Check sheet for the modelled part. Datum: model origin and axes. Units: mm. Face numbers are marked on the shaded views. A direction names the side the tool comes from. Round coordinates to 2 decimals unless told otherwise and drop trailing zeros. Order: outer loops, then holes, each group sorted by start corner. A loop starts at its lowest first (then second) coordinate and runs counter-clockwise, first axis right, second up. Notation, with made-up numbers: M 88,25.5 L 117,25.5 A19 ccw 117,47.5 Z; hole C 89,38 d10. An arc over 180 degrees is marked long. One line per item, written item: value. Start each with the question number.
(1) Cross-section at B-B, the plane y = 16. Enter the section's corners in (x, z).
(2) Release check for a two-part mould opening along Z. For the marked faces 1, 2, 3 and 4 record: released by +Z, released by -Z, zero draft, split by the parting line, or undercut.
(3) Access from +Z, -Z, +X, -X, +Y, -Y to the whole of each face (thin tool, end or side, straight path). Record for the marked faces 5, 6 and 7.
(4) Depth check by flat-ended pin: pin 1 Ø4 at (x, y) = (3, 14) entering from +Z; pin 2 Ø8 at (x, y) = (4.5, 14.5) entering from +Z. Enter the tip coordinate at first touch or a pass-through.
(5) Cross-section at A-A, the plane z = -41. Enter the section's corners in (x, y), and give its area (3 significant figures).
(6) Cross-section at C-C, the plane z = -18. Enter the section's corners in (x, y), and give its area (3 significant figures).
(7) Cross-section at D-D, the plane x = 3. Enter the section's corners in (y, z), and give its area (3 significant figures).
(8) Thickness scan on L1, parallel to X at y = 10, z = -40; L2, parallel to Y at x = -1.5, z = -62; L3, parallel to X at y = 13, z = -3. Record the ranges inside material, lowest first.
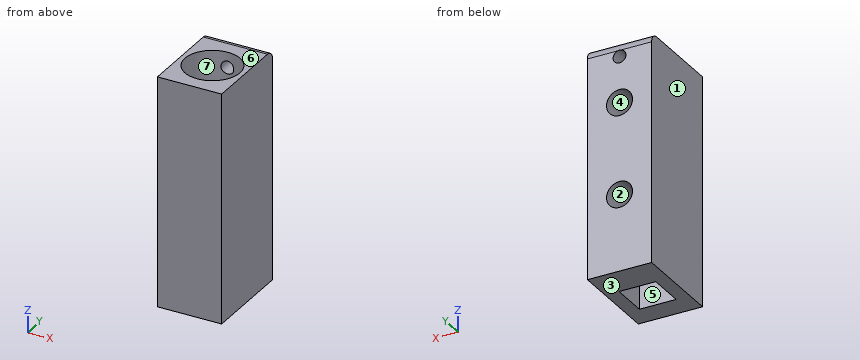
from build123d import *

# Parameters (mm, degrees)
SKETCH_1_W               = 21
SKETCH_1_H               = 30
EXTRUDE_1_DEPTH          = 75
CUT_EXTRUDE_1_DEPTH      = 82.457043894
CUT_EXTRUDE_1_DEPTH_BACK = 11
SKETCH_2_R               = 9
SKETCH_3_W               = 12
SKETCH_3_H               = 12
CUT_EXTRUDE_2_DEPTH      = 72.45802964
FILLET_1_R               = 3
HOLE_WIZARD_M5_1_REACH   = 83.457
HOLE_WIZARD_M5_1_BORE_R  = 2.1
HOLE_WIZARD_M10_1_D      = 8.5
HOLE_WIZARD_M10_1_DEPTH  = 10.5


with BuildPart() as part:
    # 草图1 → 凸台-拉伸1 (new body)
    with BuildSketch(Plane.XY):
        with Locations((0, 15)):
            Rectangle(SKETCH_1_W, SKETCH_1_H)
    extrude(amount=-EXTRUDE_1_DEPTH)

    # 草图2 → 切除-拉伸1 (cut, two sides: drawn at the far end of the back side and taken through both)
    with BuildSketch(Plane.XY.offset(-CUT_EXTRUDE_1_DEPTH_BACK)):
        with Locations(Location((0, 13.5, 0), (0, 0, 180))):
            Circle(SKETCH_2_R)
    extrude(amount=CUT_EXTRUDE_1_DEPTH + CUT_EXTRUDE_1_DEPTH_BACK, mode=Mode.SUBTRACT)

    # 草图3 → 切除-拉伸2 (cut, through all)
    with BuildSketch(Plane.XY.offset(-11)):
        with Locations((0, 13.5)):
            Rectangle(SKETCH_3_W, SKETCH_3_H)
    extrude(amount=-CUT_EXTRUDE_2_DEPTH, mode=Mode.SUBTRACT)

    # 圆角1
    fillet_1_edges = [part.edges().sort_by_distance(p)[0] for p in [
        (0, 30, 0),
    ]]
    fillet(fillet_1_edges, radius=FILLET_1_R)

    # M5 螺纹孔1 bore → M5 螺纹孔1 (cut, up to next)
    with BuildSketch(Plane(origin=(0, 30, 0), x_dir=(1, 0, 0), z_dir=(0, 1, 0)), mode=Mode.PRIVATE) as hole_wizard_m5_1_sk1:
        with Locations((0, 5)):
            Circle(HOLE_WIZARD_M5_1_BORE_R)
    hole_wizard_m5_1_tool1 = extrude(hole_wizard_m5_1_sk1.sketch, amount=-HOLE_WIZARD_M5_1_REACH, mode=Mode.PRIVATE) & part.part
    add(hole_wizard_m5_1_tool1.solids().sort_by_distance((0, 30, -5))[0], mode=Mode.SUBTRACT)

    # M10 螺纹孔1
    with Locations(Plane(origin=(0, 30, 0), x_dir=(1, 0, 0), z_dir=(0, 1, 0))):
        with Locations((0, 20), (0, 50)):
            Hole(HOLE_WIZARD_M10_1_D / 2, depth=HOLE_WIZARD_M10_1_DEPTH)


solid = part.part
Values found:
1. outline: M -10.5,-75 L -6,-75 L -6,-11 L -8.65,-11 L -8.65,0 L -10.5,0 Z; M 6,-75 L 10.5,-75 L 10.5,0 L 8.65,0 L 8.65,-11 L 6,-11 Z
2. face 1: zero draft
2. face 2: undercut
2. face 3: released by -Z
2. face 4: undercut
3. face 5: +Z, -Z
3. face 6: +Z, +X, -X, +Y, -Y
3. face 7: +Z
4. pin 1: through
4. pin 2: z = -11
5. outline: M -10.5,0 L 10.5,0 L 10.5,30 L -10.5,30 Z; hole M -6,7.5 L 6,7.5 L 6,19.5 L -6,19.5 Z
5. area: 486 mm^2
6. outline: M -10.5,0 L 10.5,0 L 10.5,30 L 3.75,30 L 3.75,19.5 L 6,19.5 L 6,7.5 L -6,7.5 L -6,19.5 L -3.75,19.5 L -3.75,30 L -10.5,30 Z
6. area: 407 mm^2
7. outline: M 0,-75 L 7.5,-75 L 7.5,-11 L 5.01,-11 L 5.01,0 L 0,0 Z; M 19.5,-75 L 30,-75 L 30,-53.01 L 19.5,-53.01 Z; M 19.5,-46.99 L 30,-46.99 L 30,-23.01 L 19.5,-23.01 Z; M 19.5,-16.99 L 30,-16.99 L 30,-3 A3 ccw 27,0 L 21.99,0 L 21.99,-11 L 19.5,-11 Z
7. area: 1,170 mm^2
8. L1: -10.5 to -6, 6 to 10.5
8. L2: 0 to 7.5, 19.5 to 30
8. L3: -10.5 to -8.99, 8.99 to 10.5
